```python
from build123d import *

# Parameters (mm, degrees)
CYLINDER002_R          = 2.5
CYLINDER002_DEPTH      = 10
CYLINDER001_R          = 2.5
CYLINDER001_DEPTH      = 10
CYLINDER_R             = 2.5
CYLINDER_DEPTH         = 10
BOX_W                  = 176
BOX_H                  = 25
BOX_DEPTH              = 3
CHAMFER_SIZE           = 2
FILLET_R               = 2
CYLINDER004_R          = 3
CYLINDER004_DEPTH      = 6
CYLINDER004_ROLL_ANGLE = 90
BOX003_W               = 6
BOX003_H               = 6
BOX003_DEPTH           = 15
CYLINDER003_R          = 3
CYLINDER003_DEPTH      = 6
CYLINDER003_ROLL_ANGLE = 90
BOX002_W               = 6
BOX002_H               = 6
BOX002_DEPTH           = 15
BOX001_W               = 176
BOX001_H               = 25
BOX001_DEPTH           = 3
BOX001_ROLL_ANGLE      = 90
FILLET001_R            = 2


with BuildPart() as cylinder002:
    # Cylinder002 → Cylinder002 (new body)
    with BuildSketch(Plane(origin=(88, 9, 0), x_dir=(1, 0, 0), z_dir=(0, 0, 1))):
        Circle(CYLINDER002_R)
    extrude(amount=CYLINDER002_DEPTH)


with BuildPart() as cylinder001:
    # Cylinder001 → Cylinder001 (new body)
    with BuildSketch(Plane(origin=(152, 9, 0), x_dir=(1, 0, 0), z_dir=(0, 0, 1))):
        Circle(CYLINDER001_R)
    extrude(amount=CYLINDER001_DEPTH)


with BuildPart() as cylinder:
    # Cylinder → Cylinder (new body)
    with BuildSketch(Plane(origin=(24, 9, 0), x_dir=(1, 0, 0), z_dir=(0, 0, 1))):
        Circle(CYLINDER_R)
    extrude(amount=CYLINDER_DEPTH)


with BuildPart() as fillet_body:
    # Box → Box (new body)
    with BuildSketch(Plane(origin=(0, 1, 0), x_dir=(1, 0, 0), z_dir=(0, 0, 1))):
        with Locations((88, 12.5)):
            Rectangle(BOX_W, BOX_H)
    extrude(amount=BOX_DEPTH)

    # Cut: cut Cylinder
    add(cylinder.part, mode=Mode.SUBTRACT)

    # Cut001: cut Cylinder001
    add(cylinder001.part, mode=Mode.SUBTRACT)

    # Cut002: cut Cylinder002
    add(cylinder002.part, mode=Mode.SUBTRACT)

    # Chamfer
    chamfer_edges = [fillet_body.edges().sort_by_distance(p)[0] for p in [
        (85.5, 9, 3),
        (21.5, 9, 3),
        (149.5, 9, 3),
    ]]
    chamfer(chamfer_edges, length=CHAMFER_SIZE)

    # Fillet
    fillet_edges = [fillet_body.edges().sort_by_distance(p)[0] for p in [
        (0, 1, 1.5),
        (176, 1, 1.5),
    ]]
    fillet(fillet_edges, radius=FILLET_R)


with BuildPart() as cylinder004:
    # Cylinder004 → Cylinder004 (new body)
    with BuildSketch(Plane.XY):
        Circle(CYLINDER004_R)
    extrude(amount=CYLINDER004_DEPTH)


with BuildPart() as cylinder004_1:
    # Cylinder004 roll: moved
    add(cylinder004.part.rotate(Axis((0, 0, 0), (1, 0, 0)), CYLINDER004_ROLL_ANGLE))


with BuildPart() as cylinder004_2:
    # Cylinder004 placement: moved
    add(cylinder004_1.part.moved(Location((36, 6, 0))))


with BuildPart() as fusion001:
    # Box003 → Box003 (new body)
    with BuildSketch(Plane(origin=(33, 0, 0), x_dir=(1, 0, 0), z_dir=(0, 0, 1))):
        with Locations((3, 3)):
            Rectangle(BOX003_W, BOX003_H)
    extrude(amount=BOX003_DEPTH)

    # Fusion001: union Cylinder004
    add(cylinder004_2.part)


with BuildPart() as fusion001_1:
    # Fusion001 placement: moved
    add(fusion001.part.moved(Location((103, 22, 11))))


with BuildPart() as cylinder003:
    # Cylinder003 → Cylinder003 (new body)
    with BuildSketch(Plane.XY):
        Circle(CYLINDER003_R)
    extrude(amount=CYLINDER003_DEPTH)


with BuildPart() as cylinder003_1:
    # Cylinder003 roll: moved
    add(cylinder003.part.rotate(Axis((0, 0, 0), (1, 0, 0)), CYLINDER003_ROLL_ANGLE))


with BuildPart() as cylinder003_2:
    # Cylinder003 placement: moved
    add(cylinder003_1.part.moved(Location((36, 6, 0))))


with BuildPart() as fusion:
    # Box002 → Box002 (new body)
    with BuildSketch(Plane(origin=(33, 0, 0), x_dir=(1, 0, 0), z_dir=(0, 0, 1))):
        with Locations((3, 3)):
            Rectangle(BOX002_W, BOX002_H)
    extrude(amount=BOX002_DEPTH)

    # Fusion: union Cylinder003
    add(cylinder003_2.part)


with BuildPart() as fusion_1:
    # Fusion placement: moved
    add(fusion.part.moved(Location((1, 22, 11))))


with BuildPart() as f_4u_ears:
    # Box001 → Box001 (new body)
    with BuildSketch(Plane.XY):
        with Locations((88, 12.5)):
            Rectangle(BOX001_W, BOX001_H)
    extrude(amount=BOX001_DEPTH)


with BuildPart() as f_4u_ears_1:
    # Box001 roll: moved
    add(f_4u_ears.part.rotate(Axis((0, 0, 0), (1, 0, 0)), BOX001_ROLL_ANGLE))


with BuildPart() as f_4u_ears_2:
    # Box001 placement: moved
    add(f_4u_ears_1.part.moved(Location((0, 26, 0))))

    # Cut003: cut Fusion
    add(fusion_1.part, mode=Mode.SUBTRACT)

    # Cut004: cut Fusion001
    add(fusion001_1.part, mode=Mode.SUBTRACT)

    # Fillet001
    fillet001_edges = [f_4u_ears_2.edges().sort_by_distance(p)[0] for p in [
        (0, 24.5, 25),
        (176, 24.5, 25),
    ]]
    fillet(fillet001_edges, radius=FILLET001_R)

    # Fusion002: union Fillet body
    add(fillet_body.part)


solid = f_4u_ears_2.part
```
The listing builds one solid part. Answer for the finished solid, in the listing's coordinates (mm). A direction names the side the tool comes from. Round coordinates to 2 decimals unless told otherwise and drop trailing zeros. Order: outer loops, then holes, each group sorted by start corner. A loop starts at its lowest first (then second) coordinate and runs counter-clockwise, first axis right, second up. Notation, with made-up numbers: (70.5, 77) -> (107.5, 77) arc R17 cw to (107.5, 86) -> close; hole circle Ø10 at (15, 33). An arc over 180 degrees is marked (long way). Answer as CSV lines item,"result".
Q1. Given pin 1 (1.5 mm diameter, centred on x = 39, z = 11, fed in from +Y); pin 2 (3 mm diameter, centred on x = 95, y = 18, fed in from +Z), each flat-ended and moving along its own axis, determine where each tip first touches the part or whether it passes through.
Computed values:
pin 1,"passes through"
pin 2,"stops at z = 3"
Q2. A cutting plane is placed at D-D on x = 109. Determine the outline of the cut face in (y, z).
Computed values:
outline,"(1, 0) -> (26, 0) -> (26, 25) -> (23, 25) -> (23, 3) -> (1, 3) -> close"
Q3. Which of the six approach directions +Z, -Z, +X, -X, +Y, -Y give full straight-line access (tool end or side, diameter ignored) to faces 4 (the flat face through (87, 26, 13)), 5 (the flat face through (136, 24, 18))?
Computed values:
face 4,"+Z, -Z, +X, -X, +Y"
face 5,"+Z, +Y, -Y"
Q4. For a pull along Y with two mould halves and no side action, classify faces 1 (the flat face through (87, 23, 14)), 2 (the cylindrical face through (86, 7.5, 0.5)), 3 (the flat face through (158, 25, 25)) as +Y half, -Y half, draft (parallel to the pull), parting line (faces both ways), or undercut.
Computed values:
face 1,"-Y half"
face 2,"undercut"
face 3,"draft"
Q5. A cutting plane is placed at B-B on z = 15.5. Determine the outline of the cut face in (x, y), plus the area to 3 significant figures.
Computed values:
outline,"(0, 23) -> (34, 23) -> (34, 26) -> (0, 26) -> close; (40, 23) -> (136, 23) -> (136, 26) -> (40, 26) -> close; (142, 23) -> (176, 23) -> (176, 26) -> (142, 26) -> close"
area,"492 mm^2"
Q6. Consider line 1 (X direction, y = 9, z = 0.3); line 2 (X direction, y = 23.75, z = 17); line 3 (Y direction, x = 88, z = 0.7). Determine where each line is inside the solid, lowest interval first. Write a range as from..to.
Computed values:
line 1,"x = 0..21.5, 26.5..85.5, 90.5..149.5, 154.5..176"
line 2,"x = 0..34, 40..136, 142..176"
line 3,"y = 1..6.5, 11.5..26"
Q7. A cutting plane is placed at C-C on x = 152. Determine the outline of the cut face in (y, z).
Computed values:
outline,"(1, 0) -> (6.5, 0) -> (6.5, 1) -> (4.5, 3) -> (1, 3) -> close; (11.5, 0) -> (26, 0) -> (26, 25) -> (23, 25) -> (23, 3) -> (13.5, 3) -> (11.5, 1) -> close"
Q8. A cutting plane is placed at A-A on y = 9. Determine the outline of the cut face in (x, z), plus the area to 3 significant figures.
Computed values:
outline,"(0, 0) -> (21.5, 0) -> (21.5, 1) -> (19.5, 3) -> (0, 3) -> close; (26.5, 0) -> (85.5, 0) -> (85.5, 1) -> (83.5, 3) -> (28.5, 3) -> (26.5, 1) -> close; (90.5, 0) -> (149.5, 0) -> (149.5, 1) -> (147.5, 3) -> (92.5, 3) -> (90.5, 1) -> close; (154.5, 0) -> (176, 0) -> (176, 3) -> (156.5, 3) -> (154.5, 1) -> close"
area,"471 mm^2"
